Model file for the job. Use its own axes, mm. A direction names the side the tool comes from. Round coordinates to 2 decimals unless told otherwise and drop trailing zeros. Loops run counter-clockwise (first coordinate to the right, second up) from the corner with the lowest first, then second, coordinate; pieces in that order, holes last. Notation, with made-up numbers: (-40, 29.5) - (-32, 29.5) arc R30 ccw to (-32, 58.5) - close; hole circle Ø6 at (-2.5, 27.5). An arc over 180 degrees is marked (long way). Answer as a JSON object with one key per item and string values.
from build123d import *

# Parameters (mm, degrees)
SKETCH1_R               = 12.5
BOSS_EXTRUDE1_DEPTH     = 3
SKETCH2_R               = 8
BOSS_EXTRUDE2_DEPTH     = 96
SKETCH5_R               = 1.5
CUT_EXTRUDE1_DEPTH      = 13.5
CUT_EXTRUDE1_DEPTH_BACK = 13.5
SCALE1_SCALE            = 2


with BuildPart() as part:
    # Sketch1 → Boss-Extrude1 (new body, symmetric)
    with BuildSketch(Plane(origin=(0, 0, 0), x_dir=(1, 0, 0), z_dir=(0, 1, 0))):
        Circle(SKETCH1_R)
    extrude(amount=BOSS_EXTRUDE1_DEPTH, both=True)

    # Sketch2 → Boss-Extrude2 (add)
    with BuildSketch(Plane(origin=(0, 3, 0), x_dir=(1, 0, 0), z_dir=(0, 1, 0))):
        Circle(SKETCH2_R)
    extrude(amount=BOSS_EXTRUDE2_DEPTH)

    # Sketch5 → Cut-Extrude1 (cut, two sides)
    with BuildSketch(Plane(origin=(0, 0, 0), x_dir=(0, 0, -1), z_dir=(1, 0, 0))) as cut_extrude1_sk:
        with Locations((0, 92)):
            Circle(SKETCH5_R)
    extrude(amount=CUT_EXTRUDE1_DEPTH, mode=Mode.SUBTRACT)
    extrude(cut_extrude1_sk.sketch, amount=-CUT_EXTRUDE1_DEPTH_BACK, mode=Mode.SUBTRACT)


with BuildPart() as part_1:
    # Scale1: scaled about (-2.171e-06, 44.005415619, -5.482e-06)
    add(part.part.scale(SCALE1_SCALE).moved(Location((2.171e-06, -44.005415619, 5.482e-06))))


solid = part_1.part
1) Probe probe 1 along Y at (x, z) = (1, 16.5); probe 2 along Z at (x, y) = (-1, 138.5); probe 3 along X at (y, z) = (36, 11). List the from-to ranges inside material, lowest first.
Values follow:
{"probe 1": "-50.01 to -38.01", "probe 2": "-15.97 to -2.6, 2.6 to 15.97", "probe 3": "-11.62 to 11.62"}
2) Tool access for faces 1 (the flat face through (0, 153.995, 0)), 2 (the cylindrical face through (14.78, 56.65, 6.13)): list every direction of +Z, -Z, +X, -X, +Y, -Y with a clear straight run to the whole face (end or side of a thin tool).
Values follow:
{"face 1": "+Z, -Z, +X, -X, +Y", "face 2": "+Y"}
3) Drop flat-ended pins along their axis: P1, Ø1.5, axis at y = -4.5, z = 2.5, coming from the +X side; P2, Ø1.5, axis at x = 18.5, y = 2, coming from the -Z side; P3, Ø1, axis at x = 1.5, y = 58.5, coming from the -Z side; P4, Ø3, axis at x = 11.5, y = 82, coming from the -Z side. Give the stop position or say it passes through.
Values follow:
{"P1": "x = 15.9", "P2": "through", "P3": "z = -15.97", "P4": "z = -12.49"}
4) Slice it at C-C on y = 64.5. List the corners of the cut face in (x, z).
Values follow:
{"outline": "circle Ø32 at (0, 0)"}
5) Slice it at A-A on x = -8. List the corners of the cut face in (y, z).
Values follow:
{"outline": "(-50.01, -23.69) - (-38.01, -23.69) - (-38.01, -13.86) - (153.99, -13.86) - (153.99, 13.86) - (-38.01, 13.86) - (-38.01, 23.69) - (-50.01, 23.69) - close; hole circle Ø6 at (139.99, 0)"}
6) Slice it at B-B on z = -10.5. List the corners of the cut face in (x, y), then the cut area to 3 significant figures.
Values follow:
{"outline": "(-22.69, -50.01) - (22.69, -50.01) - (22.69, -38.01) - (12.07, -38.01) - (12.07, 153.99) - (-12.07, 153.99) - (-12.07, -38.01) - (-22.69, -38.01) - close", "area": "5,180 mm²"}
7) Slice it at D-D on x = 5.5. List the corners of the cut face in (y, z), then the cut area to 3 significant figures.
Values follow:
{"outline": "(-50.01, -24.39) - (-38.01, -24.39) - (-38.01, -15.02) - (153.99, -15.02) - (153.99, 15.02) - (-38.01, 15.02) - (-38.01, 24.39) - (-50.01, 24.39) - close; hole circle Ø6 at (139.99, 0)", "area": "6,330 mm²"}
